Verification items for the finished model (mm, model axes). A direction names the side the tool comes from. Coordinates: 2 decimals unless noted, no trailing zeros. Write each loop counter-clockwise with the first axis right and the second up, starting at its lowest first coordinate (ties: lowest second). Pieces come first, ordered by that corner, then holes. Notation, with made-up numbers: (45, 82.5) - (77, 82.5) arc R13 cw to (77, 89.5) - close; hole circle Ø4 at (-23.75, -36). An arc over 180 degrees is marked (long way). Answer as CSV lines item,"result". Start each with the question number.
```python
from build123d import *

# Parameters (mm, degrees)
SKETCH_W        = 80
SKETCH_H        = 60
PAD_DEPTH       = 30
POCKET_DEPTH    = 30
SKETCH003_W     = 30
SKETCH003_H     = 16
PAD001_DEPTH    = 30
POCKET001_DEPTH = 60
SKETCH005_R     = 5
HOLE_DEPTH      = 16
SKETCH006_R     = 8
HOLE001_DEPTH   = 16


with BuildPart() as part:
    # Sketch → Pad (new body)
    with BuildSketch(Plane.XY):
        with Locations((40, 30)):
            Rectangle(SKETCH_W, SKETCH_H)
    extrude(amount=PAD_DEPTH)

    # Sketch001 (on Face6 of Pad) → Pocket (cut)
    with BuildSketch(Plane.XY.offset(30)):
        Polygon((80, 0), (80, 35), (40, 0), align=None)
    extrude(amount=-POCKET_DEPTH, mode=Mode.SUBTRACT)

    # Sketch003 (on Face4 of Pocket) → Pad001 (join)
    with BuildSketch(Plane.XY.offset(30)):
        with Locations((15, 8)):
            Rectangle(SKETCH003_W, SKETCH003_H)
        with Locations((15, 52)):
            Rectangle(SKETCH003_W, SKETCH003_H)
    extrude(amount=PAD001_DEPTH)

    # Sketch004 (on Face7 of Pad001) → Pocket001 (cut)
    with BuildSketch(Plane(origin=(0, 60, 0), x_dir=(-1, 0, 0), z_dir=(0, 1, 0))):
        Polygon((-30, 30), (-80, 14), (-80, 30), align=None)
    extrude(amount=-POCKET001_DEPTH, mode=Mode.SUBTRACT)

    # Sketch005 (on Face5 of Pocket001) → Hole (cut)
    with BuildSketch(Plane.XZ):
        with Locations((15, 45)):
            Circle(SKETCH005_R)
    extrude(amount=-HOLE_DEPTH, mode=Mode.SUBTRACT)

    # Sketch006 (on Face17 of Hole) → Hole001 (cut)
    with BuildSketch(Plane.XZ.offset(-44)):
        with Locations((15, 45)):
            Circle(SKETCH006_R)
    extrude(amount=-HOLE001_DEPTH, mode=Mode.SUBTRACT)


solid = part.part
```
1. Draft check along Z on faces 4 (the face through (18, 8, 49)), 5 (the face through (30, 52, 45)), 6 (the face through (13.959, 51.888, 52.932)), 7 (the face through (15, 52, 60)). Enter one of: pulls with the +Z half, pulls with the -Z half, needs draft (parallel to the pull), parting line crosses it, or undercut.
2. Cross-section at A-A (x = 15). Record the cut outline in (y, z).
3. Depth check by flat-ended pin: P1, Ø5, axis at y = 51.5, z = 38, coming from the +X side; P2, Ø8, axis at x = 15, z = 45, coming from the -Y side; P3, Ø6, axis at y = 10, z = 16.5, coming from the +X side; P4, Ø3, axis at x = 62.5, y = 44.5, coming from the +Z side. Enter the tip coordinate at first touch or a pass-through.
4. Cross-section at B-B (z = 45). Record the cut outline in (x, y), and give its area (3 significant figures).
5. Scan lines: line 1 along Y through (x, z) = (24, 32.5); line 2 along Z through (x, y) = (15, 11.5); line 3 along Z through (x, y) = (15, 51). Record each from-to range of solid material in increasing order. Write a range as from..to.
6. Access from +Z, -Z, +X, -X, +Y, -Y to the whole of each face (thin tool, end or side, straight path). Record for faces 1 (the face through (8, 44, 38)), 2 (the face through (39, 30, 0)), 3 (the face through (30, 8, 45)).
7. Cross-section at C-C (y = 21). Record the cut outline in (x, z), and give its area (3 significant figures).
8. Cross-section at D-D (y = 9). Record the cut outline in (x, z), and give its area (3 significant figures).
Completed:
1,face 4,"undercut"
1,face 5,"needs draft"
1,face 6,"undercut"
1,face 7,"pulls with the +Z half"
2,outline,"(0, 0) - (60, 0) - (60, 37) - (44, 37) - (44, 30) - (16, 30) - (16, 40) - (0, 40) - close; (0, 50) - (16, 50) - (16, 60) - (0, 60) - close; (44, 53) - (60, 53) - (60, 60) - (44, 60) - close"
3,P1,"stops at x = 30"
3,P2,"passes through"
3,P3,"stops at x = 54.86"
3,P4,"stops at z = 20.08"
4,outline,"(0, 0) - (10, 0) - (10, 16) - (0, 16) - close; (0, 44) - (7, 44) - (7, 60) - (0, 60) - close; (20, 0) - (30, 0) - (30, 16) - (20, 16) - close; (23, 44) - (30, 44) - (30, 60) - (23, 60) - close"
4,area,"544 mm2"
5,line 1,"y = 0..16, 44..60"
5,line 2,"z = 0..40, 50..60"
5,line 3,"z = 0..37, 53..60"
6,face 1,"+Z, +X, -X"
6,face 2,"-Z, +X, -X, +Y, -Y"
6,face 3,"+Z, +X, +Y, -Y"
7,outline,"(0, 0) - (64, 0) - (64, 19.12) - (30, 30) - (0, 30) - close"
7,area,"1,740 mm2"
8,outline,"(0, 0) - (50.29, 0) - (50.29, 23.51) - (30, 30) - (30, 60) - (0, 60) - close; hole circle Ø10 at (15, 45)"
8,area,"2,260 mm2"
